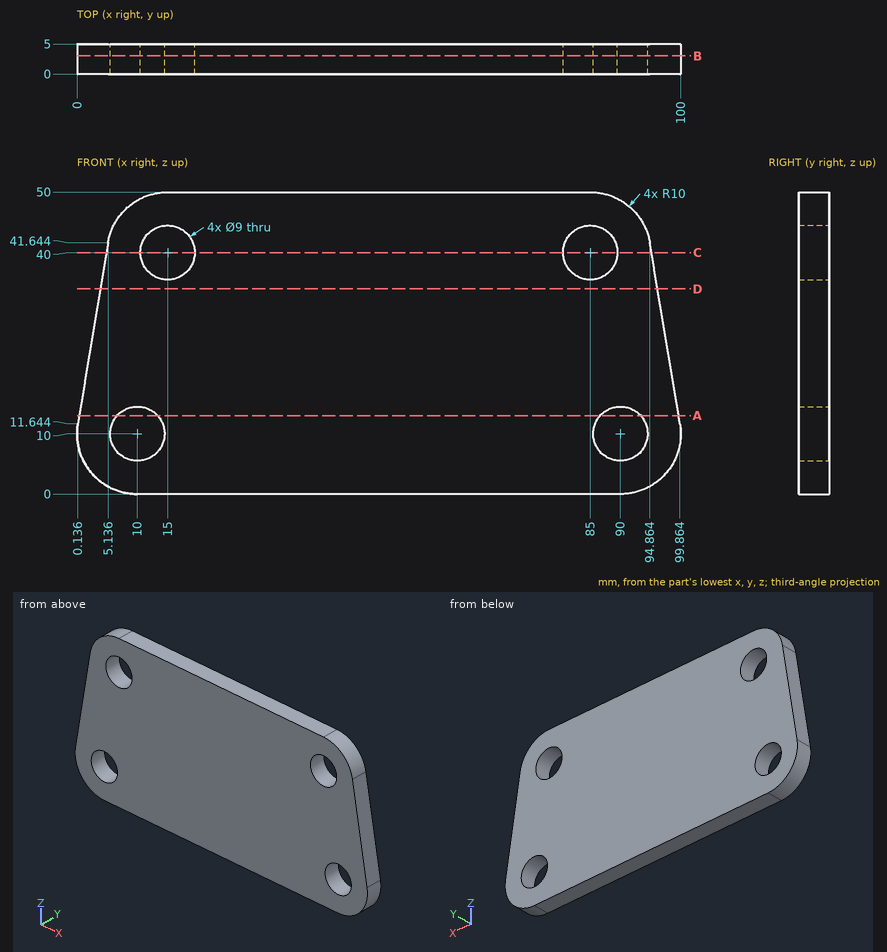
Check sheet for the drawn part. Datum: minimum x, y, z corner. Units: mm. Give positions to 0.01 mm unless a question says otherwise; leave off trailing zeros. Order: outer loops, then holes, each group sorted by start corner. A loop starts at its lowest first (then second) coordinate and runs counter-clockwise, first axis right, second up. Notation, with made-up numbers: (2.5, 8.5) - (7.5, 8.5) arc R14 cw to (7.5, 12.5) - close; hole circle Ø1 at (14.25, 46.25). An arc over 180 degrees is marked (long way). Answer in a Markdown table with one row per item. Add a question column.
Q1. Cross-section at D-D, the plane z = 34. Enter the section's corners in (x, y), then the cut area to 3 significant figures.
Q2. Gauge pin test, flat ends, axial feed: pin 1 (5.5 mm diameter, centred on x = 15, z = 40, fed in from +Y); pin 2 (1 mm diameter, centred on y = 2, z = 17.5, fed in from +X). Record the tip position at first contact, or that the pin passes through.
Q3. Cross-section at C-C, the plane z = 40. Enter the section's corners in (x, y).
Q4. Material ranges on probe 1 along X at (y, z) = (3.25, 10); probe 2 along X at (y, z) = (2.35, 40); probe 3 along Z at (x, y) = (85, 1.9), recorded low to high. Write a range as from..to.
Q5. Cross-section at B-B, the plane y = 3.05. Enter the section's corners in (x, z), then the cut area to 3 significant figures.
Q6. Cross-section at A-A, the plane z = 13. Enter the section's corners in (x, y), then the cut area to 3 significant figures.
Check values:
| question | item | result |
|---|---|---|
| 1 | outline | (3.86, 0) - (96.14, 0) - (96.14, 5) - (3.86, 5) - close |
| 1 | area | 461 mm^2 |
| 2 | pin 1 | passes through |
| 2 | pin 2 | stops at x = 98.97 |
| 3 | outline | (4.86, 0) - (10.5, 0) - (10.5, 5) - (4.86, 5) - close; (19.5, 0) - (80.5, 0) - (80.5, 5) - (19.5, 5) - close; (89.5, 0) - (95.14, 0) - (95.14, 5) - (89.5, 5) - close |
| 4 | probe 1 | x = 0..5.5, 14.5..85.5, 94.5..100 |
| 4 | probe 2 | x = 4.86..10.5, 19.5..80.5, 89.5..95.14 |
| 4 | probe 3 | z = 0..35.5, 44.5..50 |
| 5 | outline | (0.14, 11.64) arc R10 ccw to (10, 0) - (90, 0) arc R10 ccw to (99.86, 11.64) - (94.86, 41.64) arc R10 ccw to (85, 50) - (15, 50) arc R10 ccw to (5.14, 41.64) - close; hole circle Ø9 at (10, 10); hole circle Ø9 at (15, 40); hole circle Ø9 at (85, 40); hole circle Ø9 at (90, 10) |
| 5 | area | 4,420 mm^2 |
| 6 | outline | (0.36, 0) - (6.65, 0) - (6.65, 5) - (0.36, 5) - close; (13.35, 0) - (86.65, 0) - (86.65, 5) - (13.35, 5) - close; (93.35, 0) - (99.64, 0) - (99.64, 5) - (93.35, 5) - close |
| 6 | area | 429 mm^2 |
